Print and shaded views of the part. All mm, measured from the part's lowest x, y and z. A direction names the side the tool comes from. Give positions to 0.01 mm unless a question says otherwise; leave off trailing zeros. Loops run counter-clockwise (first coordinate to the right, second up) from the corner with the lowest first, then second, coordinate; pieces in that order, holes last.
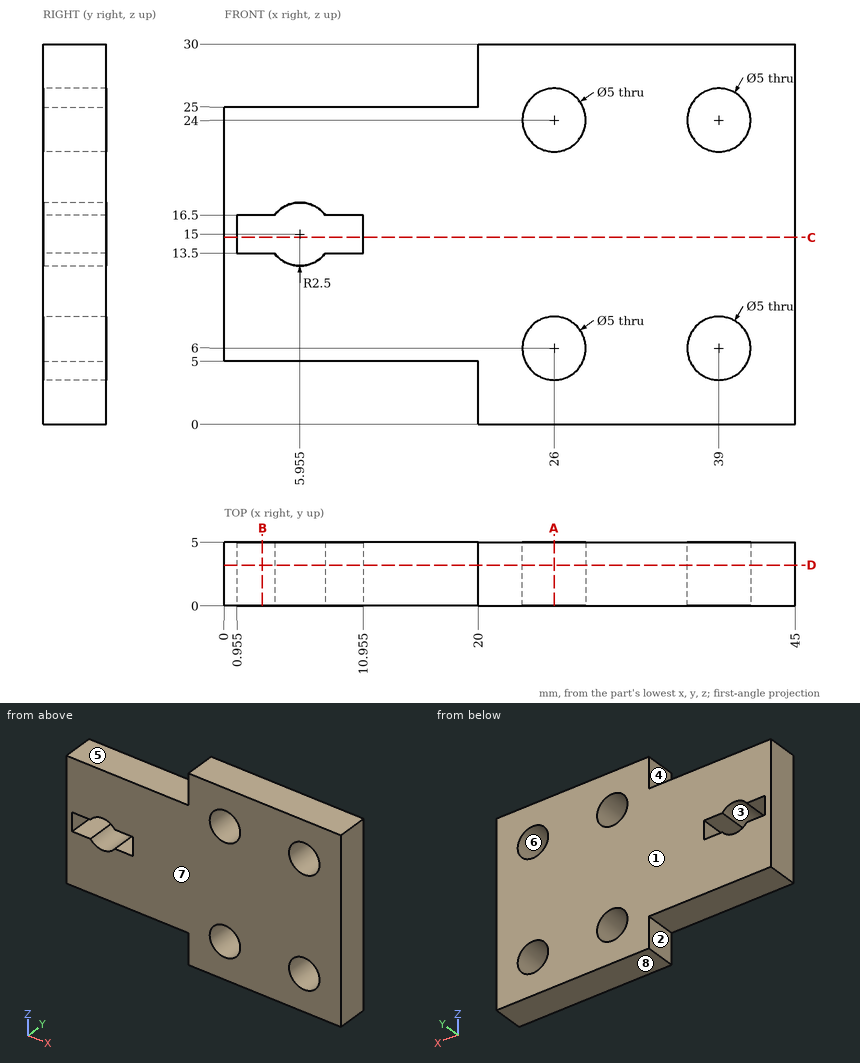
1. Saw through at B-B, the plane x = 3. List the corners of the cut face in (y, z), and give its area (3 significant figures).
Responses:
outline: (0, 5) - (5, 5) - (5, 13.5) - (0, 13.5) - close; (0, 16.5) - (5, 16.5) - (5, 25) - (0, 25) - close
area: 85.0 mm2
2. Pull direction Z, two halves, no side cores. Call the marked faces 5, 6, 7 and 8: released by +Z, released by -Z, zero draft, split by the parting line, or undercut.
Responses:
face 5: released by +Z
face 6: undercut
face 7: zero draft
face 8: released by -Z
3. Drop flat-ended pins along their axis: pin 1 (1.5 mm diameter, centred on x = 5, y = 2.5, fed in from +Z); pin 2 (4 mm diameter, centred on x = 39, z = 6, fed in from +Y); pin 3 (2.5 mm diameter, centred on y = 2, z = 26.5, fed in from -X); pin 4 (0.9 mm diameter, centred on x = 2.5, y = 3.5, fed in from -Z). Give the stop position or say it passes through.
Responses:
pin 1: stops at z = 25
pin 2: passes through
pin 3: stops at x = 20
pin 4: stops at z = 5
4. Saw through at C-C, the plane z = 14.75. List the corners of the cut face in (x, y) (1 decimal), and give its area (3 significant figures).
Responses:
outline: (0, 0) - (1, 0) - (1, 5) - (0, 5) - close; (11, 0) - (45, 0) - (45, 5) - (11, 5) - close
area: 175 mm2
5. Tool access for the marked faces 1, 2, 3 and 4: list every direction of +Z, -Z, +X, -X, +Y, -Y with a clear straight run to the whole face (end or side of a thin tool).
Responses:
face 1: +Z, -Z, +X, -X, +Y
face 2: -Z, -X, +Y, -Y
face 3: +Y, -Y
face 4: +Z, -X, +Y, -Y
6. Probe line 1 along X through (y, z) = (2.1, 24); line 2 along Z through (x, y) = (39, 1.9); line 3 along Z through (x, y) = (37.5, 4.4). List the from-to ranges inside material, lowest first.
Responses:
line 1: x = 0 to 23.5, 28.5 to 36.5, 41.5 to 45
line 2: z = 0 to 3.5, 8.5 to 21.5, 26.5 to 30
line 3: z = 0 to 4, 8 to 22, 26 to 30
7. Saw through at A-A, the plane x = 26. List the corners of the cut face in (y, z).
Responses:
outline: (0, 0) - (5, 0) - (5, 3.5) - (0, 3.5) - close; (0, 8.5) - (5, 8.5) - (5, 21.5) - (0, 21.5) - close; (0, 26.5) - (5, 26.5) - (5, 30) - (0, 30) - close
8. Saw through at D-D, the plane y = 3.2. List the corners of the cut face in (x, z) (1 decimal).
Responses:
outline: (0, 5) - (20, 5) - (20, 0) - (45, 0) - (45, 30) - (20, 30) - (20, 25) - (0, 25) - close; hole (1, 13.5) - (4, 13.5) arc R2.5 ccw to (8, 13.5) - (11, 13.5) - (11, 16.5) - (8, 16.5) arc R2.5 ccw to (4, 16.5) - (1, 16.5) - close; hole circle Ø5 at (26, 6); hole circle Ø5 at (26, 24); hole circle Ø5 at (39, 6); hole circle Ø5 at (39, 24)
